Read the model definition and answer for the solid it produces. Units are mm, in the model's axes. A direction names the side the tool comes from. Coordinates: 2 decimals unless noted, no trailing zeros. Loops run counter-clockwise (first coordinate to the right, second up) from the corner with the lowest first, then second, coordinate; pieces in that order, holes last. Notation, with made-up numbers: (-28.5, 72.5) -> (0.5, 72.5) arc R25 ccw to (0.5, 101.5) -> close; hole circle Ø1 at (-23, 50). An arc over 180 degrees is marked (long way). Answer as a JSON object with one key per item and string values. Group by question number.
Q1. The part is cut by section C-C on z = 4.5. Write down the section's boundary in (x, y), and give its area (3 significant figures).
Q2. The part is cut by section D-D on z = -29.5. Write down the section's boundary in (x, y).
Q3. Straight lines are drawn through the part: line 1 along Z through (x, y) = (0, 3.25); line 2 along X through (y, z) = (42, 30); line 3 along X through (y, z) = (20.5, -26.5). For each, find the intervals that lie inside material, in ascending order. Write a range as [from, to].
Q4. Each of these flat-tipped pins is pushed along its axis until it touches: P1, Ø2, axis at x = -27, z = -15.5, coming from the +Y side; P2, Ø4, axis at y = 25.5, z = -8, coming from the -X side; P3, Ø10.5, axis at x = 2, z = 0, coming from the -Y side. Where does it stop, or does it pass through?
Q5. For faces 4 (the cylindrical face through (-8.21, 2.46, -6.3)), 5 (the flat face through (0, 60, 0)), 6 (the flat face through (-2.5, 35, 0)), determine the directions among +Z, -Z, +X, -X, +Y, -Y from which every point of the face is accessible in a straight line to the end or side of a thin tool.
Q6. The part is cut by section B-B on x = 0. Write down the section's boundary in (y, z), and give its area (3 significant figures).
Q7. Determine the mould class of faces 1 (the flat face through (0, 5, 0)), 2 (the cylindrical face through (-4.88, 29.58, -37.18)), 3 (the flat face through (8, 0, 8)) for opening direction Z: released by +Z, released by -Z, zero draft, split by the parting line, or undercut.
Q8. The part is cut by section A-A on y = 15. Write down the section's boundary in (x, z), and give its area (3 significant figures).
from build123d import *

# Parameters (mm, degrees)
SKETCH1_R           = 37.5
BOSS_EXTRUDE1_DEPTH = 60
CUT_EXTRUDE1_DEPTH  = 50
SKETCH3_R           = 10.35
CUT_EXTRUDE2_DEPTH  = 5


with BuildPart() as part:
    # Sketch1 → Boss-Extrude1 (new body)
    with BuildSketch(Plane(origin=(0, 0, 0), x_dir=(1, 0, 0), z_dir=(0, 1, 0))):
        Circle(SKETCH1_R)
    extrude(amount=BOSS_EXTRUDE1_DEPTH)

    # Sketch2 → Cut-Extrude1 (cut)
    with BuildSketch(Plane(origin=(0, 60, 0), x_dir=(1, 0, 0), z_dir=(0, 1, 0))):
        with BuildLine():
            Line((-2.5, -32.403703492), (-2.5, 32.403703492))
            ThreePointArc((-2.5, 32.403703492), (-32.5, 0), (-2.5, -32.403703492))
        make_face()
        with BuildLine():
            ThreePointArc((32.5, 0), (23.848480035, 22.079402166), (2.5, 32.403703492))
            Line((2.5, 32.403703492), (2.5, -32.403703492))
            ThreePointArc((2.5, -32.403703492), (23.848480035, -22.079402166), (32.5, 0))
        make_face()
    extrude(amount=-CUT_EXTRUDE1_DEPTH, mode=Mode.SUBTRACT)

    # Sketch3 → Cut-Extrude2 (cut)
    with BuildSketch(Plane.XZ):
        Circle(SKETCH3_R)
    extrude(amount=-CUT_EXTRUDE2_DEPTH, mode=Mode.SUBTRACT)


solid = part.part
Final values:
{
 "1": {"outline": "(-37.23, 0) -> (-9.32, 0) -> (-9.32, 5) -> (9.32, 5) -> (9.32, 0) -> (37.23, 0) -> (37.23, 60) -> (32.19, 60) -> (32.19, 10) -> (2.5, 10) -> (2.5, 60) -> (-2.5, 60) -> (-2.5, 10) -> (-32.19, 10) -> (-32.19, 60) -> (-37.23, 60) -> close", "area": "1,410 mm2"},
 "2": {"outline": "(-23.15, 0) -> (23.15, 0) -> (23.15, 60) -> (13.64, 60) -> (13.64, 10) -> (2.5, 10) -> (2.5, 60) -> (-2.5, 60) -> (-2.5, 10) -> (-13.64, 10) -> (-13.64, 60) -> (-23.15, 60) -> close"},
 "3": {"line 1": "z = [-37.5, -10.35], [10.35, 37.5]", "line 2": "x = [-22.5, -12.5], [-2.5, 2.5], [12.5, 22.5]", "line 3": "x = [-26.53, -18.81], [-2.5, 2.5], [18.81, 26.53]"},
 "4": {"P1": "stops at y = 10", "P2": "stops at x = -37.02", "P3": "stops at y = 5"},
 "5": {"face 4": "-Y", "face 5": "+Z, -Z, +X, -X, +Y", "face 6": "+Y"},
 "6": {"outline": "(0, -37.5) -> (60, -37.5) -> (60, 37.5) -> (0, 37.5) -> (0, 10.35) -> (5, 10.35) -> (5, -10.35) -> (0, -10.35) -> close", "area": "4,400 mm2"},
 "7": {"face 1": "undercut", "face 2": "split by the parting line", "face 3": "zero draft"},
 "8": {"outline": "circle Ø75 at (0, 0); hole (-2.5, -32.4) -> (-2.5, 32.4) arc R32.5 ccw to start; hole (2.5, -32.4) arc R32.5 ccw to (2.5, 32.4) -> close", "area": "1,420 mm2"}
}
